Can you work these out from the model? Positions are in its coordinate system, mm. A direction names the side the tool comes from. Coordinates: 2 decimals unless noted, no trailing zeros. Write each loop counter-clockwise with the first axis right and the second up, starting at its lowest first coordinate (ties: lowest second). Pieces come first, ordered by that corner, then holes.
```python
from build123d import *

# Parameters (mm, degrees)
SKETCH1_R           = 1.6
BOSS_EXTRUDE1_DEPTH = 2


with BuildPart() as part:
    # Sketch1 → Boss-Extrude1 (new body)
    with BuildSketch(Plane(origin=(0, 0, 0), x_dir=(1, 0, 0), z_dir=(0, 1, 0))):
        with BuildLine():
            Line((6.185029122, 11), (22.5, 11))
            ThreePointArc((22.5, 11), (24.621320344, 10.121320344), (25.5, 8))
            Line((25.5, 8), (25.5, -8))
            ThreePointArc((25.5, -8), (24.621320344, -10.121320344), (22.5, -11))
            Line((22.5, -11), (-22.5, -11))
            ThreePointArc((-22.5, -11), (-24.621320344, -10.121320344), (-25.5, -8))
            Line((-25.5, -8), (-25.5, 8))
            ThreePointArc((-25.5, 8), (-24.621320344, 10.121320344), (-22.5, 11))
            Line((-22.5, 11), (-6.185029122, 11))
            Line((-6.185029122, 11), (-2.912197092, 20.279508432))
            ThreePointArc((-2.912197092, 20.279508432), (0, 24), (2.912197092, 20.279508432))
            Line((2.912197092, 20.279508432), (6.185029122, 11))
        make_face()
        with Locations(Location((-22.5, 8, 0), (0, 0, 270))):
            Circle(SKETCH1_R, mode=Mode.SUBTRACT)
        with Locations(Location((-22.5, -8, 0), (0, 0, 270))):
            Circle(SKETCH1_R, mode=Mode.SUBTRACT)
        with Locations(Location((22.5, -8, 0), (0, 0, 270))):
            Circle(SKETCH1_R, mode=Mode.SUBTRACT)
        with Locations(Location((22.5, 8, 0), (0, 0, 270))):
            Circle(SKETCH1_R, mode=Mode.SUBTRACT)
        with Locations(Location((0, 21, 0), (0, 0, 270))):
            Circle(SKETCH1_R, mode=Mode.SUBTRACT)
        with BuildLine():
            Line((-0.487430468, 18.039862919), (-2.28542798, 11))
            Line((-2.28542798, 11), (2.28542798, 11))
            Line((2.28542798, 11), (0.487430468, 18.039862919))
            ThreePointArc((0.487430468, 18.039862919), (0, 18), (-0.487430468, 18.039862919))
        make_face(mode=Mode.SUBTRACT)
        with BuildLine():
            Line((-19.5, -8), (19.5, -8))
            ThreePointArc((19.5, -8), (20.378679656, -5.878679656), (22.5, -5))
            Line((22.5, -5), (22.5, 5))
            ThreePointArc((22.5, 5), (20.378679656, 5.878679656), (19.5, 8))
            Line((19.5, 8), (-19.5, 8))
            ThreePointArc((-19.5, 8), (-20.378679656, 5.878679656), (-22.5, 5))
            Line((-22.5, 5), (-22.5, -5))
            ThreePointArc((-22.5, -5), (-20.378679656, -5.878679656), (-19.5, -8))
        make_face(mode=Mode.SUBTRACT)
    extrude(amount=BOSS_EXTRUDE1_DEPTH)


solid = part.part
```
1. If we section it at D-D, the plane x = 1: List the corners of the cut face in (y, z) for me, plus the area to 3 significant figures.
2. If we section it at A-A, the plane z = 0: List the corners of the cut face in (x, y) for me, plus the area to 3 significant figures.
3. If I drill on L1, parallel to Z at x = -17.5, y = 1.15; L2, parallel to X at y = 1.3, z = -1.5; L3, parallel to X at y = 0.75, z = 7, over which ranges is the centre line in solid material (lowest first)?
4. We'd pull the mould along X, two halves only. Please class faces 3 (the face through (-25.5, 1, 0)), 4 (the face through (0, 1, -8)), 5 (the face through (24.6, 0.99, -10.14)): released by +X, released by -X, zero draft, split by the parting line, or undercut.
5. Which directions (+Z, -Z, +X, -X, +Y, -Y) give clear straight access to the entire face, cutting with the end or side of a thin tool? Please do faces 1 (the face through (-20.36, 0.99, -5.9)), 2 (the face through (24.64, 0.99, 10.1)).
6. If we section it at C-C, the plane y = 0.35: Count the separate pieces of the cut face and the enclosed holes in it, plus the area to 3 significant figures.
7. If we section it at B-B, the plane x = -17.5: List the corners of the cut face in (y, z) for me, plus the area to 3 significant figures.
8. I'm going to push a flat-ended pin straight in: P1, Ø1, axis at x = 15, y = 1, coming from the -Z side. Where does the tip first touch, or does it pass through?
Answers:
1. outline: (0, -23.83) - (2, -23.83) - (2, -22.25) - (0, -22.25) - close; (0, -19.75) - (2, -19.75) - (2, -16.03) - (0, -16.03) - close; (0, -11) - (2, -11) - (2, -8) - (0, -8) - close; (0, 8) - (2, 8) - (2, 11) - (0, 11) - close
1. area: 22.6 mm2
2. outline: (-25.5, 0) - (-22.5, 0) - (-22.5, 2) - (-25.5, 2) - close; (22.5, 0) - (25.5, 0) - (25.5, 2) - (22.5, 2) - close
2. area: 12.0 mm2
3. L1: z = -11 to -8, 8 to 11
3. L2: x = -25.5 to -22.5, 22.5 to 25.5
3. L3: x = -25.5 to -23.75, -21.25 to -19.67, 19.67 to 21.25, 23.75 to 25.5
4. face 3: released by -X
4. face 4: undercut
4. face 5: released by +X
5. face 1: +Y, -Y
5. face 2: +Z, +X, +Y, -Y
6. separate pieces: 1
6. enclosed holes: 7
6. area: 466 mm2
7. outline: (0, -11) - (2, -11) - (2, -8) - (0, -8) - close; (0, 8) - (2, 8) - (2, 11) - (0, 11) - close
7. area: 12.0 mm2
8. P1: stops at z = -11
